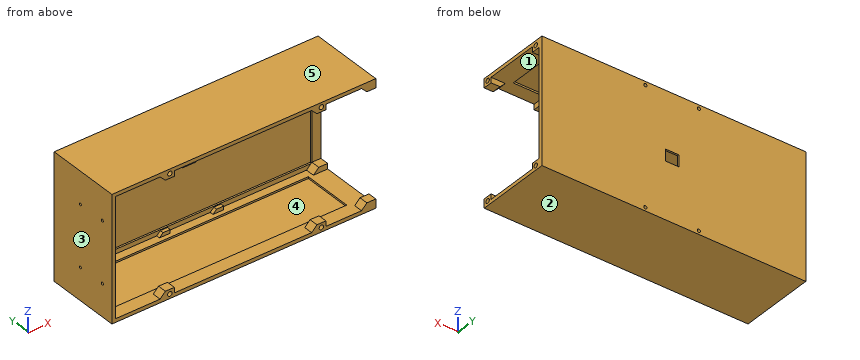
Autodesk Inventor part; units mm, degrees
ref_plane "YZ Plane" through (0, 0, 0) normal (1, 0, 0) x (0, 1, 0)
ref_plane "XZ Plane" through (0, 0, 0) normal (0, 1, 0) x (-1, 0, 0)
ref_plane "XY Plane" through (0, 0, 0) normal (0, 0, 1) x (1, 0, 0)
sketch "Sketch1" plane through (0, 0, 0) normal (0, 1, 0) x (-1, 0, 0)
  line L0 (146, -66) -> (-146, -66)
  line L1 (-146, -66) -> (-146, 66) construction
  line L2 (-146, 66) -> (146, 66)
  line L3 (146, 66) -> (146, -66)
  line L4 (146, 0) -> (-146, 0) construction
  line L5 (0, 66) -> (0, -66) construction
  line L6 (150, -70) -> (-146, -70)
  line L7 (-146, 70) -> (150, 70)
  line L8 (150, 70) -> (150, -70)
  line L9 (-146, 66) -> (-146, 70)
  line L10 (-146, -66) -> (-146, -70)
  point P0 (0, 0)
  point P1 (0, 0)
  dimension "d0" = 292
  dimension "d1" = 132
  dimension "d2" = 4
  dimension "d3" = 4
extrude "Extrusion1" add sketch "Sketch1" along normal blind 80
sketch "Sketch2" plane through (0, 0, 0) normal (0, -1, 0) x (1, 0, 0)
  line L0 (146, 66) -> (-146, 66) construction
  line L1 (-146, -66) -> (146, -66) construction
  line L2 (146, 66) -> (146, -66) construction
  line L3 (146, 0) -> (-146, 0) construction
  line L4 (-146, 66) -> (-146, -66) construction
  line L5 (-90, 66) -> (-90, 60)
  line L6 (-90, 60) -> (-80, 60)
  line L7 (-80, 60) -> (-80, 66)
  line L8 (-90, -66) -> (-90, -60)
  line L9 (-90, -60) -> (-80, -60)
  line L10 (-80, -60) -> (-80, -66)
  line L11 (0, 66) -> (0, -66) construction
  line L12 (90, 66) -> (90, 60)
  line L13 (90, 60) -> (80, 60)
  line L14 (80, 60) -> (80, 66)
  line L15 (80, -60) -> (80, -66)
  line L16 (90, -60) -> (80, -60)
  line L17 (90, -66) -> (90, -60)
  line L18 (-90, 66) -> (-80, 66)
  line L19 (-80, -66) -> (-90, -66)
  line L20 (90, -66) -> (80, -66)
  line L21 (80, 66) -> (90, 66)
  point P0 (0, 0)
  dimension "d6" = 6
  dimension "d7" = 56
  dimension "d8" = 10
extrude "Extrusion2" add sketch "Sketch2" against normal blind 10
sketch "Sketch3" plane through (-150, 0, -70) normal (-1, 0, 0) x (0, 0, 1)
  line L0 (136, 10) -> (130, 10) construction
  line L1 (10, 10) -> (4, 10) construction
  line L2 (10, 10) -> (4, 10) construction
  line L3 (130, 10) -> (136, 10) construction
  line L4 (10, 10) -> (130, 10) construction
  line L5 (136, 80) -> (4, 80) construction
  line L6 (70, 80) -> (70, 0) construction
  line L7 (0, 0) -> (140, 0) construction
  line L8 (0, 0) -> (0, 80) construction
  line L9 (0, 14) -> (140, 14) construction
  circle A0 centre (36, 14) radius 1.5
  circle A1 centre (104, 14) radius 1.5
  line L10 (0, 0) -> (0, 80) construction
  line L11 (0, 46) -> (140, 46) construction
  line L12 (140, 0) -> (140, 80) construction
  circle A2 centre (36, 46) radius 1.5
  circle A3 centre (104, 46) radius 1.5
  dimension "d11" = 4
  dimension "d12" = 3
  dimension "d13" = 68
  dimension "d26" = 32
  dimension "d27" = 3
extrude "Extrusion3" cut sketch "Sketch3" against normal blind 10
sketch "Sketch4" plane through (0, 0, 0) normal (0, -1, 0) x (1, 0, 0)
  line L0 (146, 66) -> (-146, 66)
  line L1 (146, 66) -> (136, 66)
  line L2 (136, 66) -> (136, 60)
  line L3 (136, 60) -> (146, 60)
  line L4 (146, 60) -> (146, 66)
  line L5 (146, -66) -> (146, -70) construction
  line L6 (146, -66) -> (146, 66) construction
  line L7 (146, 0) -> (-146, 0) construction
  line L8 (-146, 66) -> (-146, -66) construction
  line L9 (146, -66) -> (136, -66)
  line L10 (136, -66) -> (136, -60)
  line L11 (136, -60) -> (146, -60)
  line L12 (146, -60) -> (146, -66)
  point P0 (0, 0)
  dimension "d16" = 10
  dimension "d17" = 6
extrude "Extrusion4" add sketch "Sketch4" against normal blind 10
sketch "Sketch6" plane through (146, 0, 70) normal (1, 0, 0) x (0, 0, -1)
  line L0 (4, 0) -> (4, 80) construction
  line L1 (136, 10) -> (136, 80) construction
  line L2 (4, 80) -> (136, 80) construction
  line L3 (4, 0) -> (10, 0) construction
  line L4 (130, 0) -> (130, 10) construction
  line L5 (10, 0) -> (130, 0) construction
  line L6 (140, 80) -> (0, 80) construction
  line L7 (70, 80) -> (70, 0) construction
  line L8 (4, 80) -> (10, 80)
  line L9 (10, 80) -> (10, 70)
  line L10 (10, 70) -> (4, 70)
  line L11 (4, 70) -> (4, 80)
  line L12 (136, 0) -> (136, 80) construction
  line L13 (136, 80) -> (4, 80) construction
  line L14 (0, 80) -> (140, 80) construction
  line L15 (136, 80) -> (130, 80)
  line L16 (130, 80) -> (130, 70)
  line L17 (130, 70) -> (136, 70)
  line L18 (136, 70) -> (136, 80)
  dimension "d20" = 10
extrude "Extrusion5" add sketch "Sketch6" against normal blind 10
sketch "Sketch7" plane through (146, 0, 70) normal (1, 0, 0) x (0, 0, -1)
  line L0 (0, 80) -> (10, 80) construction
  line L1 (10, 70) -> (4, 70) construction
  line L2 (0, 80) -> (10, 70) construction
  line L3 (10, 80) -> (0, 70) construction
  line L4 (0, 0) -> (0, 80) construction
  line L5 (0, 40) -> (140, 40) construction
  line L6 (140, 0) -> (140, 80) construction
  line L7 (70, 0) -> (70, 80) construction
  line L8 (140, 80) -> (0, 80) construction
  circle A0 centre (5, 75) radius 2.5
  circle A1 centre (135, 75) radius 2.5
  circle A2 centre (5, 5) radius 2.5
  circle A3 centre (135, 5) radius 2.5
  dimension "d23" = 5
extrude "Extrusion6" cut sketch "Sketch7" against normal blind 6
sketch "Sketch8" plane through (0, 80, 0) normal (0, 1, 0) x (1, 0, 0)
  line L0 (146, 70) -> (146, 60)
  line L1 (-150, 70) -> (-150, -70)
  line L2 (146, 70) -> (-150, 70)
  line L3 (-150, 70) -> (-150, -70)
  line L4 (-150, -70) -> (146, -70)
  line L5 (146, -70) -> (146, 70)
  point P0 (0, 0)
extrude "Extrusion7" add sketch "Sketch8" along normal blind 4
sketch "Sketch11" plane through (0, 0, 0) normal (0, -1, 0) x (1, 0, 0)
  circle A0 centre (85, 65) radius 2.5
  line L0 (-150, 70) -> (146, 70)
  line L1 (90, 60) -> (90, 66)
  line L2 (80, 66) -> (-80, 66)
  line L3 (0, 66) -> (0, -66) construction
  line L4 (-80, -66) -> (80, -66)
  circle A1 centre (-85, 65) radius 2.5
  line L5 (146, 60) -> (136, 60) construction
  line L6 (146, 60) -> (146, -60) construction
  line L7 (146, 60) -> (146, -60) construction
  line L8 (146, 0) -> (-146, 0) construction
  line L9 (-146, 66) -> (-146, -66) construction
  circle A2 centre (85, -65) radius 2.5
  circle A3 centre (-85, -65) radius 2.5
  point P0 (0, 0)
  dimension "d39" = 5
  dimension "d40" = 5
  dimension "d41" = 5
extrude "Extrusion8" cut sketch "Sketch11" against normal blind 6
sketch "Sketch12" plane through (-90, 0, 60) normal (-1, 0, 0) x (0, 0, 1)
  line L0 (6, 0) -> (0, 0)
  line L1 (6, 10) -> (6, 0)
  line L2 (0, 10) -> (6, 10)
  line L3 (0, 0) -> (0, 10)
  line L4 (-120, 0) -> (-126, 0)
  line L5 (-120, 0) -> (-120, 10)
  line L6 (-126, 10) -> (-120, 10)
  line L7 (-126, 0) -> (-126, 10)
  point P0 (-60, 0)
  point P1 (10, 84)
extrude "Extrusion9" add sketch "Sketch12" along normal blind 6
sketch "Sketch13" plane through (80, 0, 60) normal (-1, 0, 0) x (0, 0, 1)
  line L0 (6, 0) -> (0, 0)
  line L1 (6, 10) -> (6, 0)
  line L2 (0, 10) -> (6, 10)
  line L3 (0, 0) -> (0, 10)
  line L4 (-120, 0) -> (-126, 0)
  line L5 (-120, 0) -> (-120, 10)
  line L6 (-126, 10) -> (-120, 10)
  line L7 (-126, 0) -> (-126, 10)
  point P0 (-60, 0)
extrude "Extrusion10" add sketch "Sketch13" along normal blind 6
sketch "Sketch14" plane through (136, 0, 60) normal (-1, 0, 0) x (0, 0, 1)
  line L0 (6, 0) -> (0, 0)
  line L1 (6, 10) -> (6, 0)
  line L2 (0, 10) -> (6, 10)
  line L3 (0, 0) -> (0, 10)
  line L4 (-120, 0) -> (-126, 0)
  line L5 (-120, 0) -> (-120, 10)
  line L6 (-126, 10) -> (-120, 10)
  line L7 (-126, 0) -> (-126, 10)
  line L8 (0, 70) -> (6, 70)
  line L9 (6, 80) -> (6, 70)
  line L10 (6, 80) -> (0, 80)
  line L11 (0, 80) -> (0, 70)
  line L12 (-120, 70) -> (-120, 80)
  line L13 (-120, 80) -> (-126, 80)
  line L14 (-126, 70) -> (-126, 80)
  line L15 (-126, 70) -> (-120, 70)
  point P0 (-60, 0)
extrude "Extrusion11" add sketch "Sketch14" along normal blind 6
chamfer "Chamfer4" distance 6 angle 45 8 edges at (130, 5, 60) (130, 5, -60) (130, 75, -60) (130, 75, 60) (74, 5, 60) (74, 5, -60) (-96, 5, 60) (-96, 5, -60)
sketch "Sketch16" plane through (0, 84, 0) normal (0, 1, 0) x (1, 0, 0)
  line L0 (-30, 66) -> (30, 66) construction
  line L1 (30, 66) -> (30, -66) construction
  line L2 (30, -66) -> (-30, -66) construction
  line L3 (-30, -66) -> (-30, 66) construction
  line L4 (146, 70) -> (-150, 70) construction
  line L5 (-150, -70) -> (146, -70) construction
  line L6 (-2, 70) -> (-2, -70) construction
  line L7 (-150, 70) -> (-150, -70) construction
  line L8 (-150, 0) -> (146, 0) construction
  line L9 (146, -60) -> (146, 60) construction
  line L10 (0, 66) -> (0, -66) construction
  line L11 (-30, 0) -> (30, 0) construction
  circle A0 centre (-30, 66) radius 1.75
  circle A1 centre (30, 66) radius 1.75
  circle A2 centre (-30, -66) radius 1.75
  circle A3 centre (30, -66) radius 1.75
  line L12 (7.5, -6.5) -> (-7.5, -6.5)
  line L13 (-7.5, -6.5) -> (-7.5, 6.5)
  line L14 (-7.5, 6.5) -> (7.5, 6.5)
  line L15 (7.5, 6.5) -> (7.5, -6.5)
  line L16 (7.5, 0) -> (-7.5, 0) construction
  line L17 (0, 6.5) -> (0, -6.5) construction
  point P0 (0, 0)
  point P1 (0, 0)
  dimension "d79" = 60
  dimension "d80" = 132
  dimension "d81" = 4
  dimension "d82" = 3.5
  dimension "d85" = 15
  dimension "d86" = 13
extrude "Extrusion13" cut sketch "Sketch16" against normal blind 4
sketch "Sketch17" plane through (0, 80, 0) normal (0, -1, 0) x (1, 0, 0)
  line L0 (28.25, 66) -> (-28.25, 66)
  line L1 (-26, 66) -> (-38, 66)
  line L2 (-38, 66) -> (-38, 62)
  line L3 (-38, 62) -> (-26, 62)
  line L4 (-26, 62) -> (-26, 66)
  line L5 (0, 66) -> (0, -66) construction
  line L6 (-80, -66) -> (74, -66) construction
  line L7 (-146, 66) -> (-146, -66) construction
  line L8 (-146, 0) -> (146, 0) construction
  line L9 (146, 60) -> (146, -60) construction
  arc A0 (-31.75, 66) -> (-28.25, 66) centre (-30, 66) ccw construction
  line L10 (-30, 66) -> (-30, 62) construction
  line L11 (-28.25, 66) -> (28.25, 66)
  line L12 (28.25, -66) -> (-28.25, -66)
  line L13 (-26, -66) -> (-38, -66)
  line L14 (-38, -66) -> (-38, -62)
  line L15 (-38, -62) -> (-26, -62)
  line L16 (-26, -62) -> (-26, -66)
  arc A1 (-28.25, -66) -> (-31.75, -66) centre (-30, -66) ccw construction
  line L17 (-30, -66) -> (-30, -62) construction
  line L18 (-28.25, -66) -> (28.25, -66)
  line L19 (130, 66) -> (31.75, 66)
  line L20 (34, 66) -> (22, 66)
  line L21 (22, 66) -> (22, 62)
  line L22 (22, 62) -> (34, 62)
  line L23 (34, 62) -> (34, 66)
  line L24 (31.75, 66) -> (28.25, 66) construction
  line L25 (30, 66) -> (30, 62) construction
  line L26 (34, -66) -> (22, -66)
  line L27 (22, -66) -> (22, -62)
  line L28 (22, -62) -> (34, -62)
  line L29 (34, -62) -> (34, -66)
  line L30 (31.75, -66) -> (28.25, -66) construction
  line L31 (30, -66) -> (30, -62) construction
  point P0 (0, 0)
  point P1 (-28.25, 66)
  point P2 (31.75, 66)
  dimension "d87" = 4
  dimension "d88" = 4
  dimension "d89" = 8
  dimension "d92" = 12
  dimension "d93" = 4
  dimension "d94" = 4
extrude "Extrusion14" add sketch "Sketch17" along normal blind 4
chamfer "Chamfer5" distance 4 angle 45 4 edges at (-38, 78, 62) (22, 78, 62) (-38, 78, -62) (22, 78, -62)
sketch "Sketch18" plane through (0, 80, 0) normal (0, -1, 0) x (1, 0, 0)
  line L0 (-146, 66) -> (-146, -66) construction
  line L1 (130, 66) -> (146, 66) construction
  line L2 (-146, -66) -> (146, -66) construction
  line L3 (146, -66) -> (146, 66) construction
  line L4 (146, 66) -> (-146, 66) construction
  line L5 (-146, 66) -> (-146, -66) construction
  line L6 (136, 61) -> (-140, 61)
  line L7 (-140, 61) -> (-140, -61)
  line L8 (-140, -61) -> (136, -61)
  line L9 (136, -61) -> (136, 61)
  line L10 (146, 60) -> (146, -60) construction
  line L11 (146, 0) -> (-146, 0) construction
  line L12 (22, 66) -> (-26, 66) construction
  line L13 (-2, 66) -> (-2, -66) construction
  line L14 (-26, -66) -> (22, -66) construction
  point P0 (0, 0)
  dimension "d98" = 5
  dimension "d99" = 10
extrude "Extrusion15" cut sketch "Sketch18" against normal blind 2
sketch "Sketch19" plane through (90, 0, 66) normal (0, 0, -1) x (-1, 0, 0)
  line L0 (-35, 15) -> (231, 15)
  line L1 (231, 15) -> (231, 71)
  line L2 (231, 71) -> (-35, 71)
  line L3 (-35, 71) -> (-35, 15)
  line L4 (-40, 10) -> (-40, 0)
  line L5 (236, 0) -> (236, 80)
  line L6 (170, 10) -> (186, 10)
  line L7 (68, 76) -> (56, 76)
  point P0 (90, 0)
  dimension "d102" = 5
  dimension "d103" = 5
  dimension "d104" = 5
  dimension "d105" = 5
extrude "Extrusion16" cut sketch "Sketch19" against normal blind 2
sketch "Sketch20" plane through (-80, 0, -66) normal (0, 0, 1) x (1, 0, 0)
  line L0 (-61, 71) -> (-61, 15)
  line L1 (205, 71) -> (-61, 71)
  line L2 (205, 15) -> (205, 71)
  line L3 (-61, 15) -> (205, 15)
  point P0 (80, 0)
extrude "Extrusion18" cut sketch "Sketch20" against normal blind 2
properties part number "electronics_case"
Geometry: final body of the model. Coordinates: model frame, mm. Face numbers are marked on the shaded views. A direction names the side the tool comes from. Coordinates: 2 decimals unless noted, no trailing zeros. Loops run counter-clockwise (first coordinate to the right, second up) from the corner with the lowest first, then second, coordinate; pieces in that order, holes last. Notation, with made-up numbers: M 33.5,63 L 40.5,63 A17 ccw 40.5,72 Z; hole C 64,23.5 d11. An arc over 180 degrees is marked long. One line per item, written item: value. Start each with the question number.
1) Cut plane B-B (z = -42). Return loops of the section in (x, y), then the cut area to 3 significant figures.
2) Material intervals for L1, parallel to Y at x = -148.75, z = 34; L2, parallel to Z at x = -85, y = 2.9; L3, parallel to Z at x = -23, y = 16, sorted ascending. Write a range as from..to.
3) Cut plane C-C (y = 32). Return loops of the section in (x, z).
4) Cut plane A-A (x = -107). Return loops of the section in (y, z), then the cut area to 3 significant figures.
5) Draft query along X for the marked faces 3, 4 and 5. Return one class per face: released by +X, released by -X, zero draft, split by the parting line, or undercut.
6) Reachability of the marked faces 1 and 2 from +Z, -Z, +X, -X, +Y, -Y: full face, straight path, thin tool, end or side. Return the list, or none.
7) Pin query (flat end, axial travel): P1, Ø2.5, axis at x = 84, z = 65, coming from the -Y side; P2, Ø8, axis at y = 29, z = -29.5, coming from the +X side; P3, Ø1.5, axis at x = 81.5, z = 33.5, coming from the -Y side. Return the tip coordinate at first contact, or that it passes through.
Evaluation:
1. outline: M -150,0 L -146,0 L -146,80 L -140,80 L -140,82 L 136,82 L 136,80 L 146,80 L 146,84 L -150,84 Z
1. area: 952 mm^2
2. L1: 0..12.5, 15.5..44.5, 47.5..84
2. L2: -70..-67.5, -62.5..-60, 60..62.5, 67.5..70
2. L3: -70..-68, 68..70
3. outline: M -150,-70 L 146,-70 L 146,-66 L 125,-66 L 125,-68 L -141,-68 L -141,-66 L -146,-66 L -146,66 L -141,66 L -141,68 L 125,68 L 125,66 L 146,66 L 146,70 L -150,70 Z
4. outline: M 0,-70 L 84,-70 L 84,70 L 0,70 L 0,66 L 15,66 L 15,68 L 71,68 L 71,66 L 80,66 L 80,61 L 82,61 L 82,-61 L 80,-61 L 80,-66 L 71,-66 L 71,-68 L 15,-68 L 15,-66 L 0,-66 Z
4. area: 732 mm^2
5. face 3: released by -X
5. face 4: undercut
5. face 5: zero draft
6. face 1: none
6. face 2: -Z, +X, -X, +Y, -Y
7. P1: y = 6
7. P2: x = -146
7. P3: y = 82
